from build123d import *

# Parameters (mm, degrees)
F0_R     = 254
F1_DEPTH = 508


with BuildPart() as f1:
    # F0 (on Front) → F1 (new body)
    with BuildSketch(Plane.XZ):
        with BuildLine():
            ThreePointArc((0, 127), (37.197439, 37.197439), (127, 0))
            Line((127, 0), (1778, 0))
            Line((1778, 0), (1778, 381))
            Line((1778, 381), (2047.407684, 650.407684))
            Line((2047.407684, 650.407684), (1831.881537, 865.933831))
            Line((1831.881537, 865.933831), (1562.473853, 596.526147))
            Line((1562.473853, 596.526147), (1382.868731, 776.131269))
            Line((1382.868731, 776.131269), (1652.276414, 1045.538953))
            Line((1652.276414, 1045.538953), (1412.407684, 1285.407684))
            Line((1412.407684, 1285.407684), (1143, 1016))
            Line((1143, 1016), (889, 1016))
            Line((889, 1016), (889, 762))
            Line((889, 762), (762, 762))
            Line((762, 762), (762, 1016))
            Line((762, 1016), (381, 1016))
            ThreePointArc((381, 1016), (291.197439, 978.802561), (254, 889))
            Line((254, 889), (254, 508))
            Line((254, 508), (127, 508))
            ThreePointArc((127, 508), (37.197439, 470.802561), (0, 381))
            Line((0, 381), (0, 127))
        make_face()
        with Locations((825.5, 381)):
            Circle(F0_R, mode=Mode.SUBTRACT)
    extrude(amount=F1_DEPTH)


solid = f1.part
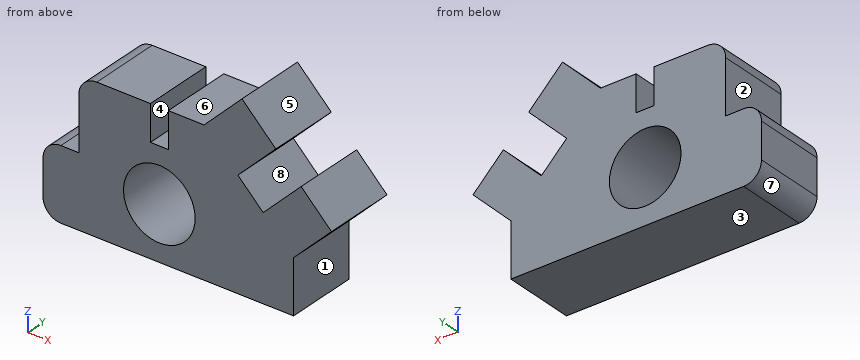
Check sheet for the modelled part. Datum: model origin and axes. Units: mm. Face numbers are marked on the shaded views. A direction names the side the tool comes from. Give positions to 0.01 mm unless a question says otherwise; leave off trailing zeros. Loops run counter-clockwise (first coordinate to the right, second up) from the corner with the lowest first, then second, coordinate; pieces in that order, holes last. Notation, with made-up numbers: M 23,14 L 46,14 A3 cw 46,19 Z; hole C 40.25,56.25 d8. An arc over 180 degrees is marked long. Use a Markdown table: item, result. Add a question column.
Q1. Mould release check, pull along X, two halves, no side actions. Record for the marked faces 6, 7 and 8: pulls with the +X half, pulls with the -X half, needs draft (parallel to the pull), parting line crosses it, or undercut.
Q2. Tool access check on the marked faces 1, 2, 3, 4 and 5. Record the directions out of +Z, -Z, +X, -X, +Y, -Y that give a thin tool (end or side, any length) a straight path to the whole face; none if there is none.
Q3. Sectioned sample at D-D, the plane x = 1189.5. Record the cut outline in (y, z), then the cut area to 3 significant figures.
Q4. Go/stop test with flat-tipped pins: pin 1 (3 mm diameter, centred on y = -232.5, z = 771, fed in from +X); pin 2 (8 mm diameter, centred on y = -268, z = 298, fed in from +X); pin 3 (1.5 mm diameter, centred on y = -297.5, z = 424.5, fed in from +X). Record where each tip stops, or that it passes through.
Q5. Sectioned sample at B-B, the plane x = 825.5. Record the cut outline in (y, z), then the cut area to 3 significant figures.
Q6. Sectioned sample at C-C, the plane z = 413. Record the cut outline in (x, y), then the cut area to 3 significant figures.
Q7. Scan lines: line 1 along Z through (x, y) = (825.5, -373.5); line 2 along X through (y, z) = (-176, 831.5); line 3 along X through (y, z) = (-33.5, 844.5). Record each from-to range of solid material in increasing order. Write a range as [from, to].
Q8. Sectioned sample at A-A, the plane y = -430. Record the cut outline in (x, z), then the cut area to 3 significant figures.
Verdict:
| question | item | result |
|---|---|---|
| 1 | face 6 | needs draft |
| 1 | face 7 | pulls with the -X half |
| 1 | face 8 | undercut |
| 2 | face 1 | -Z, +X, +Y, -Y |
| 2 | face 2 | +Z, -X, +Y, -Y |
| 2 | face 3 | -Z, +X, -X, +Y, -Y |
| 2 | face 4 | +Z, +Y, -Y |
| 2 | face 5 | +Z, +X, +Y, -Y |
| 3 | outline | M -508,0 L 0,0 L 0,1062.5 L -508,1062.5 Z |
| 3 | area | 540,000 mm^2 |
| 4 | pin 1 | x = 1928.32 |
| 4 | pin 2 | x = 1778 |
| 4 | pin 3 | x = 1822.25 |
| 5 | outline | M -508,0 L 0,0 L 0,127 L -508,127 Z; M -508,635 L 0,635 L 0,762 L -508,762 Z |
| 5 | area | 129,000 mm^2 |
| 6 | outline | M 4.1,-508 L 573.52,-508 L 573.52,0 L 4.1,0 Z; M 1077.48,-508 L 1810,-508 L 1810,0 L 1077.48,0 Z |
| 6 | area | 661,000 mm^2 |
| 7 | line 1 | [0, 127], [635, 762] |
| 7 | line 2 | [254, 762], [889, 1438.24], [1797.45, 1866.32] |
| 7 | line 3 | [254, 762], [889, 1451.24], [1810.45, 1853.32] |
| 8 | outline | M 0,127 A127 ccw 127,0 L 1778,0 L 1778,381 L 2047.41,650.41 L 1831.88,865.93 L 1562.47,596.53 L 1382.87,776.13 L 1652.28,1045.54 L 1412.41,1285.41 L 1143,1016 L 889,1016 L 889,762 L 762,762 L 762,1016 L 381,1016 A127 ccw 254,889 L 254,508 L 127,508 A127 ccw 0,381 Z; hole C 825.5,381 d508 |
| 8 | area | 1,480,000 mm^2 |
